Here's how the part is built. I have some questions about the finished solid (model axes, mm). A direction names the side the tool comes from. Coordinates: 2 decimals unless noted, no trailing zeros. Write each loop counter-clockwise with the first axis right and the second up, starting at its lowest first coordinate (ties: lowest second). Pieces come first, ordered by that corner, then holes. Notation, with made-up numbers: (-25, 76) - (-21, 76) arc R16 cw to (-21, 86) - close; hole circle Ø8 at (-17.5, 27). An arc over 180 degrees is marked (long way). Answer in a Markdown table with one row per item. Add a question column.
Item 1: We'd pull the mould along Z, two halves only. Please class faces 1 (the face through (2.85, 30.42, -3.01)), 2 (the face through (7, 30, -44)), 3 (the face through (100, 30, -25)): +Z half, -Z half, draft (parallel to the pull), parting line (faces both ways), or undercut.
Item 2: Imagine slicing it at A-A (y = 37). Please give me the cut outline in (x, z), plus the area to 3 significant figures.
Item 3: Imagine slicing it at B-B (x = 63.5). Please give me the cut outline in (y, z).
Item 4: Which directions (+Z, -Z, +X, -X, +Y, -Y) give clear straight access to the entire face, cutting with the end or side of a thin tool? Please do faces 4 (the face through (6, 30, -7)), 5 (the face through (2.85, 30.42, -46.99)).
Item 5: Imagine slicing it at C-C (z = -25). Please give me the cut outline in (x, y), plus the area to 3 significant figures.
Item 6: Imagine slicing it at D-D (y = 8.5). Please give me the cut outline in (x, z), plus the area to 3 significant figures.
Item 7: If I drill on probe 1 along X at (y, z) = (33.5, -32); probe 2 along Z at (x, y) = (61.5, 6); probe 3 along Y at (x, z) = (97.3, -25), over which ranges is the centre line in solid material (lowest first)? Write a range as from..to.
from build123d import *

# Parameters (mm, degrees)
SKETCH1_W           = 100
SKETCH1_H           = 50
BOSS_EXTRUDE1_DEPTH = 60
FILLET2_R           = 10
CUT_EXTRUDE1_DEPTH  = 80
SKETCH2_R           = 5
CUT_EXTRUDE2_DEPTH  = 127.885775404


with BuildPart() as part:
    # Sketch1 → Boss-Extrude1 (new body)
    with BuildSketch(Plane(origin=(0, 0, 0), x_dir=(1, 0, 0), z_dir=(0, 1, 0))):
        with Locations((50, 25)):
            Rectangle(SKETCH1_W, SKETCH1_H)
    extrude(amount=BOSS_EXTRUDE1_DEPTH)

    # Fillet2
    fillet2_edges = [part.edges().sort_by_distance(p)[0] for p in [
        (0, 30, -50),
        (100, 30, -50),
        (100, 30, 0),
        (0, 30, 0),
    ]]
    fillet(fillet2_edges, radius=FILLET2_R)

    # 3DSketch1 → Cut-Extrude1 (cut)
    with BuildSketch(Plane(origin=(10, 60, -5), x_dir=(0.924678098474716, 0, -0.38074980525429475), z_dir=(0, 1, 0))):
        with BuildLine():
            Line((0, 0), (73.974247878, -30.45998442))
            ThreePointArc((73.974247878, -30.45998442), (77.801073827, -30.451978543), (80.501387397, -27.740342954))
            Line((80.501387397, -27.740342954), (91.923881554, 0))
            ThreePointArc((91.923881554, 0), (91.915875677, 3.826825949), (89.204240088, 6.527139519))
            Line((89.204240088, 6.527139519), (15.22999221, 36.987123939))
            ThreePointArc((15.22999221, 36.987123939), (11.403166261, 36.979118062), (8.702852692, 34.267482473))
            Line((8.702852692, 34.267482473), (-2.719641466, 6.527139519))
            ThreePointArc((-2.719641466, 6.527139519), (-2.711635589, 2.700313569), (0, 0))
        make_face()
    extrude(amount=-CUT_EXTRUDE1_DEPTH, mode=Mode.SUBTRACT)

    # Sketch2 → Cut-Extrude2 (cut, through all)
    with BuildSketch(Plane.ZY):
        with Locations((-25, 40)):
            Circle(SKETCH2_R)
    extrude(amount=-CUT_EXTRUDE2_DEPTH, mode=Mode.SUBTRACT)


solid = part.part
Here are the results:
| question | item | result |
|---|---|---|
| 1 | face 1 | +Z half |
| 1 | face 2 | undercut |
| 1 | face 3 | draft |
| 2 | outline | (0, -40) arc R10 ccw to (10, -50) - (90, -50) arc R10 ccw to (100, -40) - (100, -29) - (95, -29) - (95, -40) arc R5 cw to (90, -45) - (10, -45) arc R5 cw to (5, -40) - (5, -29) - (0, -29) - close; (0, -21) - (5, -21) - (5, -10) arc R5 cw to (10, -5) - (90, -5) arc R5 cw to (95, -10) - (95, -21) - (100, -21) - (100, -10) arc R10 ccw to (90, 0) - (10, 0) arc R10 ccw to (0, -10) - close |
| 2 | area | 1,260 mm2 |
| 3 | outline | (0, -50) - (60, -50) - (60, -45) - (0, -45) - close; (0, -5) - (60, -5) - (60, 0) - (0, 0) - close |
| 4 | face 4 | +Y, -Y |
| 4 | face 5 | -Z, -X, +Y, -Y |
| 5 | outline | (0, 0) - (5, 0) - (5, 35) - (0, 35) - close; (0, 45) - (5, 45) - (5, 60) - (0, 60) - close; (95, 0) - (100, 0) - (100, 35) - (95, 35) - close; (95, 45) - (100, 45) - (100, 60) - (95, 60) - close |
| 5 | area | 500 mm2 |
| 6 | outline | (0, -40) arc R10 ccw to (10, -50) - (90, -50) arc R10 ccw to (100, -40) - (100, -10) arc R10 ccw to (90, 0) - (10, 0) arc R10 ccw to (0, -10) - close; hole (5, -40) arc R5 ccw to (10, -45) - (90, -45) arc R5 ccw to (95, -40) - (95, -10) arc R5 ccw to (90, -5) - (10, -5) arc R5 ccw to (5, -10) - close |
| 6 | area | 1,340 mm2 |
| 7 | probe 1 | x = 0..5, 95..100 |
| 7 | probe 2 | z = -50..-45, -5..0 |
| 7 | probe 3 | y = 0..35, 45..60 |
